Can you work these out from the model? Positions are in its coordinate system, mm. Face numbers are marked on the shaded views. A direction names the side the tool comes from. Coordinates: 2 decimals unless noted, no trailing zeros. Order: outer loops, then holes, each group sorted by start corner. A loop starts at its lowest first (then second) coordinate and runs counter-clockwise, first axis right, second up. Notation, with made-up numbers: (67, 21.5) -> (106, 21.5) arc R17 ccw to (106, 44.5) -> close; hole circle Ø5 at (48.25, 54.25). An arc over 180 degrees is marked (long way). Answer in a Markdown table with one row per item.
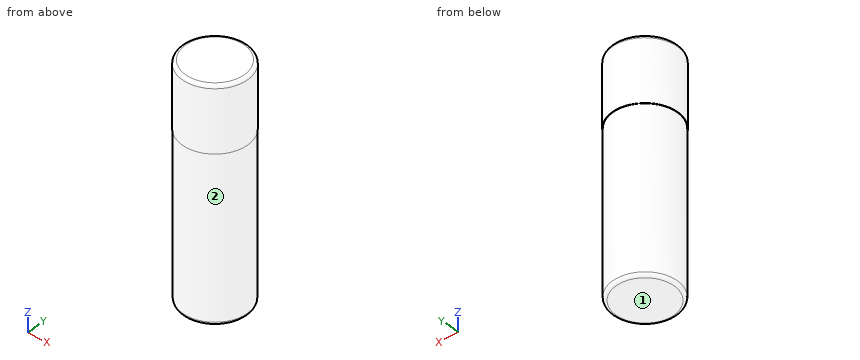
```python
from build123d import *

# Parameters (mm, degrees)
SKETCH_1_R      = 1.975
EXTRUDE_1_DEPTH = 10
FILLET_1_R      = 0.2
SKETCH_2_R      = 2
EXTRUDE_2_DEPTH = 4
FILLET_2_R      = 0.2


with BuildPart() as part:
    # 스케치1 → 보스-돌출1 (new body)
    with BuildSketch(Plane.XY):
        Circle(SKETCH_1_R)
    extrude(amount=EXTRUDE_1_DEPTH)

    # 필렛1
    fillet_1_edges = [part.edges().sort_by_distance(p)[0] for p in [
        (-1.975, 0, 0),
    ]]
    fillet(fillet_1_edges, radius=FILLET_1_R)

    # 스케치2 → 보스-돌출2 (add)
    with BuildSketch(Plane.XY.offset(10)):
        Circle(SKETCH_2_R)
    extrude(amount=EXTRUDE_2_DEPTH)

    # 필렛2
    fillet_2_edges = [part.edges().sort_by_distance(p)[0] for p in [
        (-2, 0, 14),
    ]]
    fillet(fillet_2_edges, radius=FILLET_2_R)


solid = part.part
```
(1) I need wall thicknesses on line 1 (Y direction, x = 0.05, z = 5); line 2 (X direction, y = 0.9, z = 1.75); line 3 (Y direction, x = -1, z = 3.5). Which ranges of each line are inside material? Lowest first, please. Write a range as [from, to].
Response values:
| item | result |
|---|---|
| line 1 | [-1.97, 1.97] |
| line 2 | [-1.76, 1.76] |
| line 3 | [-1.7, 1.7] |
(2) Suppose I cut it at A-A (z = 13). Please give me the cut outline in (x, y), and give its area (3 significant figures).
Response values:
| item | result |
|---|---|
| outline | circle Ø4 at (0, 0) |
| area | 12.6 mm2 |
(3) Suppose I cut it at B-B (z = 7.5). Please give me the cut outline in (x, y) (3 decimals).
Response values:
| item | result |
|---|---|
| outline | circle Ø3.95 at (0, 0) |
(4) Will these pins go through, and if not, where does the flat tip stop? pin 1 Ø1.5 at (y, z) = (-1, 3.5) entering from -X; pin 2 Ø2 at (x, z) = (1, 7) entering from +Y (3 decimals).
Response values:
| item | result |
|---|---|
| pin 1 | x = -1.96 |
| pin 2 | y = 1.975 |
(5) On a 3-axis mill with a long thin cutter (end or side, diameter ignored), from which of +Z, -Z, +X, -X, +Y, -Y can I reach the whole of each face in a straight line? I mean the marked faces 1 and 2. Say none if no direction works.
Response values:
| item | result |
|---|---|
| face 1 | -Z, +X, -X, +Y, -Y |
| face 2 | -Z |
